The model under review builds one solid part; all positions refer to its coordinate system, in mm. Give positions to 0.01 mm unless a question says otherwise; leave off trailing zeros. Write each loop counter-clockwise with the first axis right and the second up, starting at its lowest first coordinate (ties: lowest second). Pieces come first, ordered by that corner, then holes. Notation, with made-up numbers: (-2, -36.5) - (45, -36.5) arc R27 ccw to (45, -9.5) - close; hole circle Ø3 at (61.25, 55.5). An arc over 180 degrees is marked (long way). One line per question, with ' | ' between items. Start each with the question number.
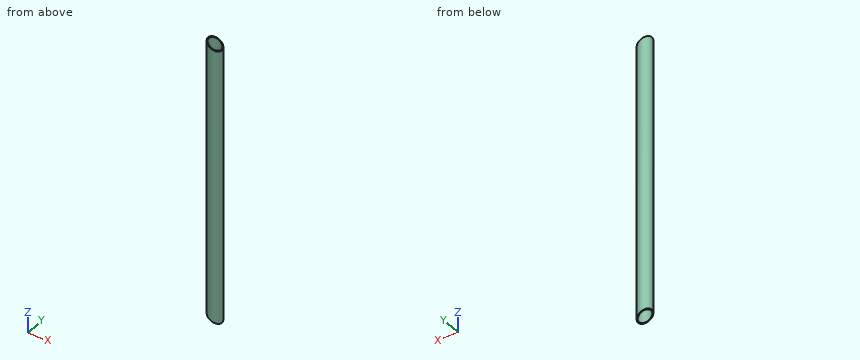
Autodesk Inventor part; units mm, degrees
ref_plane "Начальная плоскость" through (0, 0, 72.7461) normal (0, 0, 1) x (1, 0, 0)
ref_plane "Конечная плоскость" through (0, 0, 403.5678) normal (0, 0, 1) x (1, 0, 0)
ref_plane "РабПлоскость4" through (560.3889, -19.75, 75.4083) normal (0.5, 0, 0.866) x (0.866, 0, -0.5)
ref_plane "Начальная плоскость" through (0, 0, 72.7461) normal (0, 0, 1) x (1, 0, 0)
ref_plane "Конечная плоскость" through (0, 0, 403.5678) normal (0, 0, 1) x (1, 0, 0)
sketch "Эскиз" plane through (0, 0, 0) normal (0, 0, 1) x (1, 0, 0)
  circle A0 centre (0, 0) radius 7
  circle A1 centre (0, 0) radius 8
  dimension "d0" = 16
  dimension "d1" = 1
extrude "Тело" add sketch "Эскиз" along normal up to surface (330.8217 mm away) from surface at 72.7461
sketch "Sketch3" plane through (0, 0, 0) normal (0, 0, 1) x (1, 0, 0)
  line L0 (0, 0) -> (10, 0)
ref_plane "Work Plane3" through (0, 0, 0) normal (0, -1, 0) x (1, 0, 0)
sketch "Sketch4" plane through (0, 0, 0) normal (0, -1, 0) x (1, 0, 0)
  line L0 (-2, 72.7461) -> (12, 72.7461)
  line L1 (-2, 403.5678) -> (12, 403.5678)
  dimension "d7" = 330.8217
ref_plane "РабПлоскость4" through (560.3889, -19.75, 75.4083) normal (0.5, 0, 0.866) x (0.866, 0, -0.5)
split "Разделение1" plane through (560.3889, -19.75, 75.4083) removes the side toward (0.5, 0, 0.866)
ref_plane "РабПлоскость5" through (-156.5, -19.75, 167.7203) normal (-0.5, 0, -0.866) x (-0.866, 0, 0.5)
split "Разделение2" plane through (-156.5, -19.75, 167.7203) removes the side toward (-0.5, 0, -0.866)
equation "\"d0\" = G_H"
equation "\"d1\" = G_T"
equation "\"d2\" = G_L"
equation "\"G_H\" = 16"
equation "\"G_T\" = 1"
equation "\"G_L\" = d7"
equation "\"G_OFFSET_START\" = -72.74613"
equation "\"G_OFFSET_END\" = -35.21837"
equation "\"d4\" = -G_OFFSET_START"
equation "\"d5\" = G_OFFSET_END + B_L"
equation "\"B_L\" = 438.7862"
properties part number "Труба 16x1-330,82 ГОСТ 10704-91" material "Сталь, мягкая"
Item 1: Clearance check with flat-ended pins moving along their axes: P1, Ø8, axis at y = 1.5, z = 168, coming from the -X side; P2, Ø1, axis at x = 3.5, z = 259, coming from the -Y side; P3, Ø2, axis at y = -5.5, z = 286.5, coming from the -X side; P4, Ø8, axis at x = 6.5, z = 214.5, coming from the -Y side. State where each tip first meets the part, or that it passes through.
Item 2: Take a section at B-B (y = 0). Give the boundary of the cut face in (x, z), plus the area to 3 significant figures.
Item 3: Take a section at C-C (z = 192). Give the boundary of the cut face in (x, y), plus the area to 3 significant figures.
Item 4: Take a section at A-A (x = -3.75). Give the boundary of the cut face in (y, z), plus the area to 3 significant figures.
Item 5: For probe 1 along Y at (x, z) = (0, 223); probe 2 along Y at (x, z) = (2.5, 354), list the stretches that pass through material, from the lowest coordinate up.
Check sheet entries:
1) P1: stops at x = -8 | P2: stops at y = -7.42 | P3: stops at x = -6.61 | P4: stops at y = -7.6
2) outline: (-8, 81.98) - (-7, 81.41) - (-7, 402.99) - (-8, 403.57) - close; (7, 73.32) - (8, 72.75) - (8, 394.33) - (7, 394.91) - close | area: 643 mm^2
3) outline: circle Ø16 at (0, 0); hole circle Ø14 at (0, 0) | area: 47.1 mm^2
4) outline: (-7.07, 79.53) - (-5.91, 79.53) - (-5.91, 401.11) - (-7.07, 401.11) - close; (5.91, 79.53) - (7.07, 79.53) - (7.07, 401.11) - (5.91, 401.11) - close | area: 743 mm^2
5) probe 1: y = -8 to -7, 7 to 8 | probe 2: y = -7.6 to -6.54, 6.54 to 7.6
